from build123d import *

# Parameters (mm, degrees)
F1_DEPTH = 1


# Not quite as in the source:
# - ends of sketch curves that miss each other by under 0.0002 mm in the source are joined


with BuildPart() as f1:
    # F0 (on Right) → F1 (new body)
    with BuildSketch(Plane.YZ):
        with BuildLine():
            Line((137.159267, 56.359386), (94.510204, 56.359386))
            ThreePointArc((94.510204, 56.359386), (90.6662324271, 54.5568666562), (89.5937941011, 50.4489390187))
            Line((89.5937941011, 50.4489390187), (91.984617, 37.538493))
            ThreePointArc((91.984617, 37.538493), (138.4992665872, 23.165856), (185.0139164157, 37.5384923916))
            Line((185.0139164157, 37.5384923916), (187.40474, 50.448939))
            ThreePointArc((187.40474, 50.448939), (186.3323015729, 54.5568666562), (182.48833, 56.359386))
            Line((182.48833, 56.359386), (139.839267, 56.359386))
            Line((139.839267, 56.359386), (139.839267, 43.359386))
            Line((139.839267, 43.359386), (137.159267, 43.359386))
            Line((137.159267, 43.359386), (137.159267, 56.359386))
        make_face()
    extrude(amount=F1_DEPTH)


solid = f1.part
Work out the finished part from the listing and answer in its coordinate system (mm). Coordinates: 2 decimals unless noted, no trailing zeros. Write each loop counter-clockwise with the first axis right and the second up, starting at its lowest first coordinate (ties: lowest second). Pieces come first, ordered by that corner, then holes. Notation, with made-up numbers: M 50,59.5 L 64,59.5 A30 cw 64,82.5 Z; hole C 57,-23.5 d3. An arc over 180 degrees is marked long. Use one line per item in the form item = value. Start each with the question number.
1. The part is cut by section C-C (y = 111). Give the vertices of the cut face in (x, z), plus the area to 3 significant figures.
2. Straight lines are drawn through the part: probe 1 along Y at (x, z) = (0.15, 51); probe 2 along Y at (x, z) = (0.1, 47); probe 3 along Y at (x, z) = (0.5, 33). For each, find the intervals that lie inside material, in ascending order. Write a range as from..to.
3. The part is cut by section D-D (z = 41). Give the vertices of the cut face in (x, y).
4. The part is cut by section B-B (z = 51.5). Give the vertices of the cut face in (x, y).
5. The part is cut by section A-A (x = 0.7). Give the vertices of the cut face in (y, z).
Evaluation:
q1.outline = M 0,27.89 L 1,27.89 L 1,56.36 L 0,56.36 Z
q1.area = 28.5 mm^2
q2.probe_1 = 89.52..137.16, 139.84..187.48
q2.probe_2 = 90.23..137.16, 139.84..186.77
q2.probe_3 = 99.45..177.55
q3.outline = M 0,91.34 L 1,91.34 L 1,185.65 L 0,185.65 Z
q4.outline = M 0,89.51 L 1,89.51 L 1,137.16 L 0,137.16 Z; M 0,139.84 L 1,139.84 L 1,187.49 L 0,187.49 Z
q5.outline = M 89.59,50.45 L 91.98,37.54 A82.45 ccw 185.01,37.54 L 187.4,50.45 A5 ccw 182.49,56.36 L 139.84,56.36 L 139.84,43.36 L 137.16,43.36 L 137.16,56.36 L 94.51,56.36 A5 ccw Z
